Source: CAD feature listing. Evaluate the final solid. Frame: model axes, mm. Face numbers are marked on the shaded views. Give positions to 0.01 mm unless a question says otherwise; leave off trailing zeros. Order: outer loops, then holes, each group sorted by start corner. A loop starts at its lowest first (then second) coordinate and runs counter-clockwise, first axis right, second up. Notation, with made-up numbers: (-22.5, -31) -> (-0.5, -31) arc R20 ccw to (-0.5, -16) -> close; hole circle Ø10 at (41, 6.25). An arc over 180 degrees is marked (long way). Answer in a Markdown table with one row per item.
```python
from build123d import *

# Parameters (mm, degrees)
SKETCH1_R                   = 15
EXTRUDE1_DEPTH              = 200
SKETCH2_R                   = 12
CUT_EXTRUDE1_DEPTH          = 190
M6_TAPPED_HOLE2_D           = 5
M6_TAPPED_HOLE2_DEPTH       = 15
M6_TAPPED_HOLE2_CBORE_D     = 6
M6_TAPPED_HOLE2_CBORE_DEPTH = 12
M6_TAPPED_HOLE2_TIP         = 1.502151548


with BuildPart() as part:
    # Sketch1 → Extrude1 (new body)
    with BuildSketch(Plane(origin=(0, 0, 0), x_dir=(1, 0, 0), z_dir=(0, 1, 0))):
        with Locations(Location((0, 0, 0), (0, 0, 270))):
            Circle(SKETCH1_R)
    extrude(amount=-EXTRUDE1_DEPTH)

    # Sketch2 → Cut-Extrude1 (cut)
    with BuildSketch(Plane(origin=(0, 0, 0), x_dir=(1, 0, 0), z_dir=(0, 1, 0))):
        with Locations(Location((0, 0, 0), (0, 0, 270))):
            Circle(SKETCH2_R)
    extrude(amount=-CUT_EXTRUDE1_DEPTH, mode=Mode.SUBTRACT)

    # M6 Tapped Hole2
    with Locations(Plane.XZ.offset(200)):
        with Locations((0, 0)):
            CounterBoreHole(M6_TAPPED_HOLE2_D / 2, M6_TAPPED_HOLE2_CBORE_D / 2, M6_TAPPED_HOLE2_CBORE_DEPTH, depth=M6_TAPPED_HOLE2_DEPTH)
            with Locations((0, 0, -(M6_TAPPED_HOLE2_DEPTH + M6_TAPPED_HOLE2_TIP / 2))):  # 118° drill point
                Cone(0, M6_TAPPED_HOLE2_D / 2, M6_TAPPED_HOLE2_TIP, mode=Mode.SUBTRACT)


solid = part.part
```
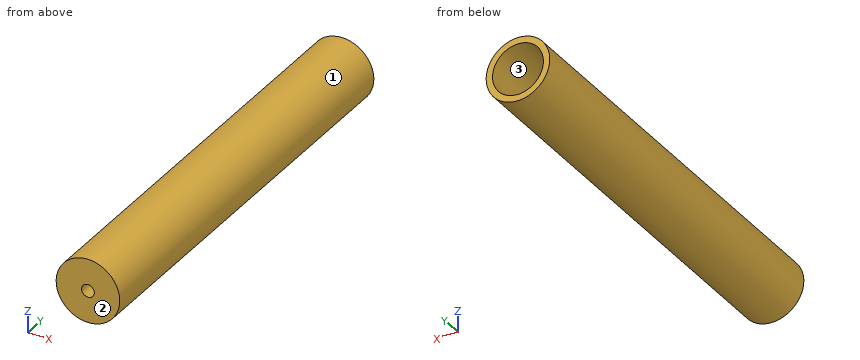
(1) Section query C-C (y = -97). Return the cut outline in (x, z), plus the area to 3 significant figures.
A:
| item | result |
|---|---|
| outline | circle Ø30 at (0, 0); hole circle Ø24 at (0, 0) |
| area | 254 mm^2 |
(2) Section query A-A (z = 0). Return the cut outline in (x, y).
A:
| item | result |
|---|---|
| outline | (-15, -200) -> (-3, -200) -> (-3, -190) -> (-12, -190) -> (-12, 0) -> (-15, 0) -> close; (3, -200) -> (15, -200) -> (15, 0) -> (12, 0) -> (12, -190) -> (3, -190) -> close |
(3) Section query B-B (x = 0). Return the cut outline in (y, z).
A:
| item | result |
|---|---|
| outline | (-200, -15) -> (0, -15) -> (0, -12) -> (-190, -12) -> (-190, -3) -> (-200, -3) -> close; (-200, 3) -> (-190, 3) -> (-190, 12) -> (0, 12) -> (0, 15) -> (-200, 15) -> close |
(4) Section query D-D (x = 10). Return the cut outline in (y, z).
A:
| item | result |
|---|---|
| outline | (-200, -11.18) -> (0, -11.18) -> (0, -6.63) -> (-190, -6.63) -> (-190, 6.63) -> (0, 6.63) -> (0, 11.18) -> (-200, 11.18) -> close |
(5) Pull-direction query (Z, two-part tool) for the marked faces 1, 2 and 3; classes: +Z half, -Z half, draft (parallel to the pull), parting line (faces both ways), or undercut.
A:
| item | result |
|---|---|
| face 1 | parting line |
| face 2 | draft |
| face 3 | undercut |
(6) Ray query, probe 1 along Z at (x, y) = (-0.75, -189.5); probe 2 along X at (y, z) = (-61, 0); probe 3 along Y at (x, z) = (5, 0). Return the intervals inside material, ascending.
A:
| item | result |
|---|---|
| probe 1 | z = -14.98 to -11.98, 11.98 to 14.98 |
| probe 2 | x = -15 to -12, 12 to 15 |
| probe 3 | y = -200 to -190 |
(7) First-contact query: pin 1 Ø4 at (x, z) = (3.5, -8) entering from +Y; pin 2 Ø3 at (x, y) = (5.5, -150) entering from -Z; pin 3 Ø3 at (x, y) = (-6.5, -54.5) entering from -Z. Flat tips, straight axial feed; report the tip coordinate or a pass-through.
A:
| item | result |
|---|---|
| pin 1 | stops at y = -190 |
| pin 2 | stops at z = -14.46 |
| pin 3 | stops at z = -14.14 |
